Verification items for this drawing (mm, ordinates from the low corner). Give positions to 0.01 mm unless a question says otherwise; leave off trailing zeros. Write each loop counter-clockwise with the first axis right and the second up, starting at its lowest first coordinate (ties: lowest second). Pieces come first, ordered by that corner, then holes. Notation, with made-up numbers: (86.5, 48) -> (109.5, 48) arc R32 ccw to (109.5, 79) -> close; hole circle Ø4 at (74.5, 74). An arc over 180 degrees is marked (long way). Write item = value, one per line.
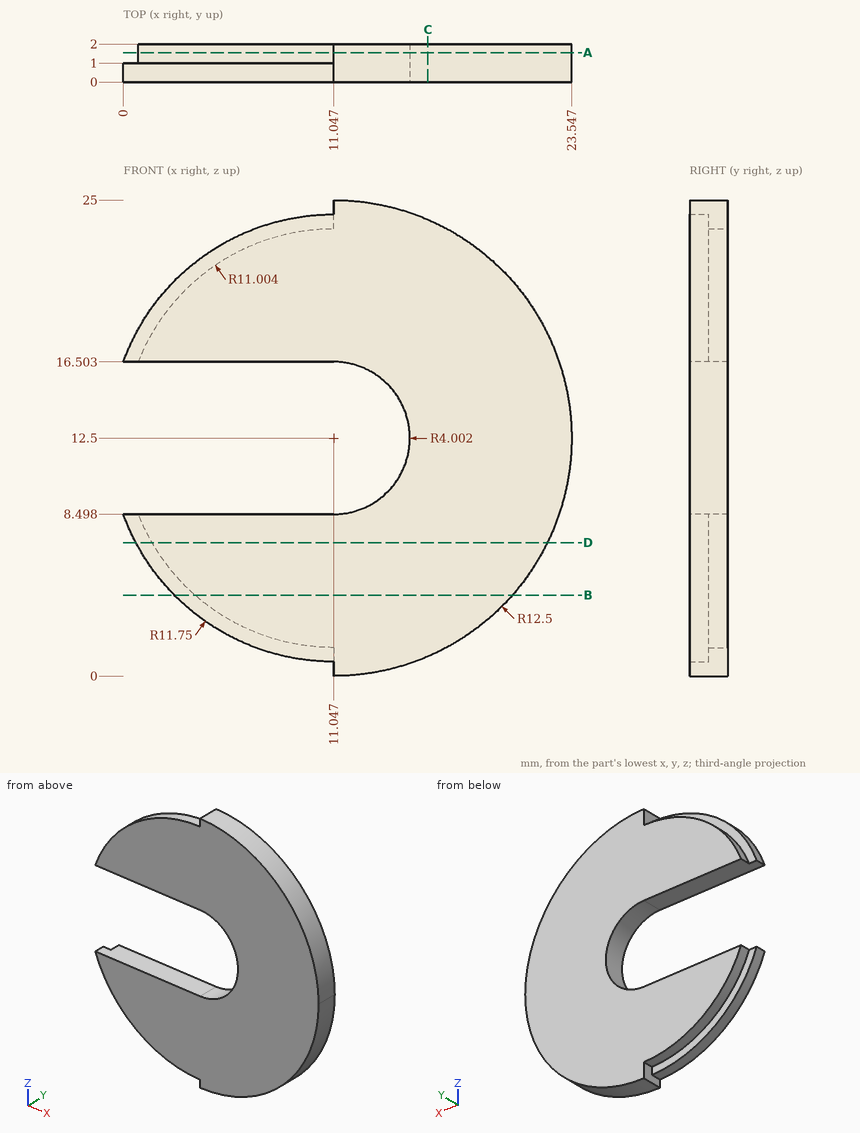
Item 1: Sectioned sample at A-A on y = 1.55. Record the cut outline in (x, z) (1 decimal).
Response values:
outline = (0.8, 8.5) arc R11 ccw to (11, 1.5) -> (11, 0) arc R12.5 ccw to (11, 25) -> (11, 23.5) arc R11 ccw to (0.8, 16.5) -> (11, 16.5) arc R4 cw to (11, 8.5) -> close
Item 2: Material ranges on line 1 (Z direction, x = 13, y = 1) (1 decimal); line 2 (Z direction, x = 12.5, y = 0.75) (1 decimal); line 3 (Z direction, x = 19.5, y = 1.1), recorded low to high.
Response values:
line_1 = 0.2 to 9, 16 to 24.8
line_2 = 0.1 to 8.8, 16.2 to 24.9
line_3 = 3.29 to 21.71
Item 3: Sectioned sample at D-D on z = 7. Record the cut outline in (x, y) (1 decimal).
Response values:
outline = (0.7, 0) -> (22.3, 0) -> (22.3, 2) -> (1.5, 2) -> (1.5, 1) -> (0.7, 1) -> close
Item 4: Sectioned sample at C-C on x = 16. Record the cut outline in (y, z).
Response values:
outline = (0, 1.02) -> (2, 1.02) -> (2, 23.98) -> (0, 23.98) -> close
Item 5: Go/stop test with flat-tipped pins: P1, Ø1, axis at x = 5.5, y = 0.5, coming from the -Z side; P2, Ø1, axis at y = 1, z = 15.5, coming from the +X side (1 decimal); P3, Ø0.6, axis at x = 3.5, y = 1.5, coming from the +Z side. Record where each tip stops, or that it passes through.
Response values:
P1 = 1.89
P2 = 23.3
P3 = 20.78
Item 6: Sectioned sample at B-B on z = 4.25. Record the cut outline in (x, y) (1 decimal).
Response values:
outline = (2.7, 0) -> (20.4, 0) -> (20.4, 2) -> (3.8, 2) -> (3.8, 1) -> (2.7, 1) -> close
